Check sheet for the modelled part. Datum: model origin and axes. Units: mm. A direction names the side the tool comes from. Coordinates: 2 decimals unless noted, no trailing zeros. Loops run counter-clockwise (first coordinate to the right, second up) from the corner with the lowest first, then second, coordinate; pieces in that order, holes last. Notation, with made-up numbers: (-34, 45) -> (17, 45) arc R6 ccw to (17, 54) -> close; hole circle Ø6 at (-39.75, 23). An arc over 180 degrees is marked (long way). Use CSV: the item, a comma, the result in double quotes.
Autodesk Inventor part; units mm, degrees
ref_plane "YZ Plane" through (0, 0, 0) normal (1, 0, 0) x (0, 1, 0)
ref_plane "XZ Plane" through (0, 0, 0) normal (0, 1, 0) x (-1, 0, 0)
ref_plane "XY Plane" through (0, 0, 0) normal (0, 0, 1) x (1, 0, 0)
sketch "Sketch2" plane through (0, 0, 0) normal (0, 1, 0) x (-1, 0, 0)
  line L0 (-40, -38) -> (40, -38)
  line L1 (40, -38) -> (40, 38)
  line L2 (40, 38) -> (-40, 38)
  line L3 (-40, 38) -> (-40, -38)
  line L4 (-40, -38) -> (40, 38) construction
  line L5 (40, -38) -> (-40, 38) construction
  point P0 (0, 0)
  dimension "d0" = 80
  dimension "d1" = 76
extrude "Extrusion1" add sketch "Sketch2" along normal blind 2.5
sketch "Sketch3" plane through (0, 2.5, 0) normal (0, 1, 0) x (1, 0, 0)
  line L0 (-35, -33) -> (35, -33)
  line L1 (35, -33) -> (35, 33)
  line L2 (35, 33) -> (-35, 33)
  line L3 (-35, 33) -> (-35, -33)
  line L4 (-35, -33) -> (35, 33) construction
  line L5 (35, -33) -> (-35, 33) construction
  line L6 (-40, 38) -> (-40, -38)
  line L7 (-40, 38) -> (-40, -38)
  line L8 (-40, -38) -> (40, -38)
  line L9 (-40, -38) -> (40, -38)
  line L10 (40, -38) -> (40, 38)
  line L11 (40, -38) -> (40, 38)
  line L12 (40, 38) -> (-40, 38)
  line L13 (40, 38) -> (-40, 38)
  point P0 (0, 0)
  dimension "d4" = 70
  dimension "d5" = 66
extrude "Extrusion2" add sketch "Sketch3" along normal blind 12.5
sketch "Sketch4" plane through (40, 0, 38) normal (1, 0, 0) x (0, 0, -1)
  line L0 (76, 0) -> (0, 0)
  line L1 (0, 0) -> (0, 15)
  line L2 (76, 0) -> (76, 15)
  line L3 (71, 2.5) -> (71, 15)
  line L4 (76, 15) -> (0, 15)
  line L5 (71, 2.5) -> (5, 2.5)
  line L6 (5, 2.5) -> (5, 15)
  line L7 (5, 15) -> (71, 15)
  line L8 (71, 15) -> (5, 15)
  line L9 (5, 2.5) -> (71, 2.5)
  line L10 (5, 2.5) -> (5, 15)
  line L11 (0, 0) -> (0, 15)
  line L12 (0, 0) -> (76, 0)
  line L13 (0, 15) -> (76, 15)
  line L14 (71, 2.5) -> (71, 15)
  line L15 (76, 0) -> (76, 15)
  line L16 (10.7, 5.15) -> (17.3, 5.15)
  line L17 (18.3, 6.15) -> (18.3, 6.85)
  line L18 (17.3, 7.85) -> (10.7, 7.85)
  line L19 (9.7, 6.85) -> (9.7, 6.15)
  line L20 (9.7, 5.15) -> (18.3, 7.85) construction
  line L21 (18.3, 5.15) -> (9.7, 7.85) construction
  arc A0 (18.3, 6.85) -> (17.3, 7.85) centre (17.3, 6.85) ccw
  arc A1 (17.3, 5.15) -> (18.3, 6.15) centre (17.3, 6.15) ccw
  arc A2 (10.7, 7.85) -> (9.7, 6.85) centre (10.7, 6.85) ccw
  arc A3 (9.7, 6.15) -> (10.7, 5.15) centre (10.7, 6.15) ccw
  point P0 (38, 0)
  point P1 (14, 6.5)
  dimension "d8" = 8.6
  dimension "d9" = 2.7
  dimension "d10" = 1
  dimension "d11" = 1
  dimension "d12" = 4
  dimension "d13" = 9
extrude "Extrusion3" cut sketch "Sketch4" against normal blind 12.5 contours A3 L19 A2 L18 A0 L17 A1 L16
fillet "Fillet1" radius 3.5 8 edges at (40, 7.5, -38) (40, 7.5, 38) (-40, 7.5, 38) (-40, 7.5, -38) (-40, 0, 0) (0, 0, -38) (40, 0, 0) (0, 0, 38)
sketch "Sketch5" plane through (0, 15, 0) normal (0, 1, 0) x (1, 0, 0)
  line L0 (36.5, 38) -> (-36.5, 38)
  line L1 (-36.5, -38) -> (36.5, -38)
  line L2 (40, -34.5) -> (40, 34.5)
  line L3 (-40, 34.5) -> (-40, -34.5)
  line L4 (35, -33) -> (-35, -33)
  line L5 (-35, -33) -> (-35, 33)
  line L6 (-35, 33) -> (35, 33)
  line L7 (35, 33) -> (35, -33)
  line L8 (-38.5, -36) -> (38.5, -36)
  line L9 (38.5, -36) -> (38.5, 36)
  line L10 (38.5, 36) -> (-38.5, 36)
  line L11 (-38.5, 36) -> (-38.5, -36)
  line L12 (-38.5, -36) -> (38.5, 36) construction
  line L13 (38.5, -36) -> (-38.5, 36) construction
  point P0 (0, 0)
  dimension "d17" = 76
  dimension "d18" = 80
  dimension "d19" = 77
  dimension "d20" = 72
extrude "Extrusion4" cut sketch "Sketch5" against normal blind 3.2
properties part number "backdoor"
1) Cross-section at D-D on z = 14. Record the boundary of the cut face in (x, y).
Answer below:
outline,"(-40, 3.5) arc R3.5 ccw to (-36.5, 0) -> (36.5, 0) arc R3.5 ccw to (40, 3.5) -> (40, 15) -> (38.5, 15) -> (38.5, 11.8) -> (35, 11.8) -> (35, 2.5) -> (-35, 2.5) -> (-35, 11.8) -> (-38.5, 11.8) -> (-38.5, 15) -> (-40, 15) -> close"
2) Draft check along Z on faces 4 (the cylindrical face through (39, 9.33, -36.95)), 5 (the flat face through (-40, 9, 0)), 6 (the flat face through (-3, 11.8, 34)), 7 (the cylindrical face through (-38.95, 9.17, 37)). Enter one of: released by +Z, released by -Z, zero draft, split by the parting line, or undercut.
Answer below:
face 4,"released by -Z"
face 5,"zero draft"
face 6,"undercut"
face 7,"released by +Z"
3) Cross-section at C-C on x = -16. Record the boundary of the cut face in (y, z), and give its area (3 significant figures).
Answer below:
outline,"(0, -34.5) arc R3.5 ccw to (3.5, -38) -> (15, -38) -> (15, -36) -> (11.8, -36) -> (11.8, -33) -> (2.5, -33) -> (2.5, 33) -> (11.8, 33) -> (11.8, 36) -> (15, 36) -> (15, 38) -> (3.5, 38) arc R3.5 ccw to (0, 34.5) -> close"
area,"291 mm²"
4) Cross-section at B-B on y = 14. Record the boundary of the cut face in (x, z), and give its area (3 significant figures).
Answer below:
outline,"(-40, -34.5) arc R3.5 ccw to (-36.5, -38) -> (36.5, -38) arc R3.5 ccw to (40, -34.5) -> (40, 34.5) arc R3.5 ccw to (36.5, 38) -> (-36.5, 38) arc R3.5 ccw to (-40, 34.5) -> close; hole (-38.5, -36) -> (38.5, -36) -> (38.5, 36) -> (-38.5, 36) -> close"
area,"525 mm²"
5) Thickness scan on line 1 along Z through (x, y) = (-33.5, 8); line 2 along X through (y, z) = (8.75, -1.5); line 3 along X through (y, z) = (13.5, 17). Record the ranges inside material, lowest first. Write a range as from..to.
Answer below:
line 1,"z = -38..-33, 33..38"
line 2,"x = -40..-35, 35..40"
line 3,"x = -40..-38.5, 38.5..40"
6) Cross-section at A-A on z = 25. Record the boundary of the cut face in (x, y), and give its area (3 significant figures).
Answer below:
outline,"(-40, 3.5) arc R3.5 ccw to (-36.5, 0) -> (36.5, 0) arc R3.5 ccw to (40, 3.5) -> (40, 5.15) -> (35, 5.15) -> (35, 2.5) -> (-35, 2.5) -> (-35, 11.8) -> (-38.5, 11.8) -> (-38.5, 15) -> (-40, 15) -> close; (35, 7.85) -> (40, 7.85) -> (40, 15) -> (38.5, 15) -> (38.5, 11.8) -> (35, 11.8) -> close"
area,"284 mm²"
7) Access from +Z, -Z, +X, -X, +Y, -Y to the whole of each face (thin tool, end or side, straight path). Record for faces 1 (the flat face through (1, 9, -38)), 2 (the flat face through (-38.5, 13, -1)), 3 (the flat face through (38, 7.85, 24)).
Answer below:
face 1,"-Z, +X, -X, +Y, -Y"
face 2,"+Y"
face 3,"+X"
8) Go/stop test with flat-tipped pins: pin 1 Ø8 at (x, z) = (17, 10) entering from +Y; pin 2 Ø1.5 at (y, z) = (2.5, -5.5) entering from +X. Record where each tip stops, or that it passes through.
Answer below:
pin 1,"stops at y = 2.5"
pin 2,"stops at x = 39.99"
